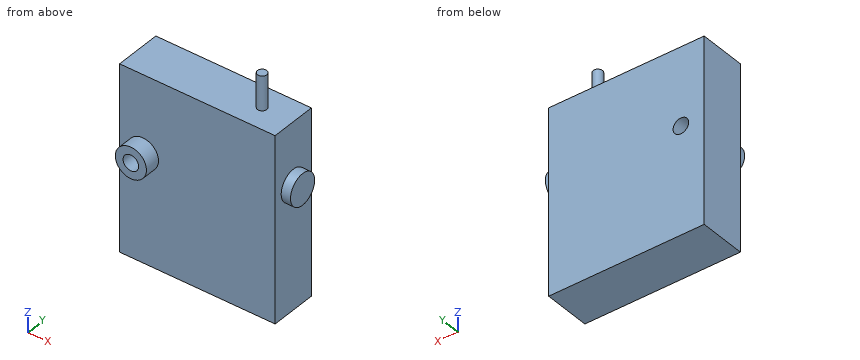
from build123d import *

# Parameters (mm, degrees)
F0_W     = 100
F0_H     = 119.065711
F1_DEPTH = 15
F2_R     = 10
F3_DEPTH = 10
F4_R     = 10
F5_DEPTH = 6
F6_R     = 3
F7_DEPTH = 22
F8_R     = 5
F9_DEPTH = 40.001


with BuildPart() as f1:
    # F0 (on Front) → F1 (new body, symmetric)
    with BuildSketch(Plane.XZ):
        with Locations((0, -3.62726)):
            Rectangle(F0_W, F0_H)
    extrude(amount=F1_DEPTH, both=True)

    # F2 (on face) → F3 (join)
    with BuildSketch(Plane.XZ.offset(15)):
        with Locations((-35, 5.905595)):
            Circle(F2_R)
    extrude(amount=F3_DEPTH)

    # F4 (on face) → F5 (join)
    with BuildSketch(Plane.YZ.offset(50)):
        with Locations((0, 15.905595)):
            Circle(F4_R)
    extrude(amount=F5_DEPTH)

    # F6 (on face) → F7 (join)
    with BuildSketch(Plane.XY.offset(55.905595)):
        with Locations((30, 0)):
            Circle(F6_R)
    extrude(amount=F7_DEPTH)

    # F8 (on face) → F9 (cut, through all)
    with BuildSketch(Plane.XZ.offset(25)):
        with Locations((-35, 5.905595)):
            Circle(F8_R)
    extrude(amount=-F9_DEPTH, mode=Mode.SUBTRACT)


solid = f1.part
Source: CAD feature listing. Evaluate the final solid. Frame: model axes, mm. Coordinates: 2 decimals unless noted, no trailing zeros. Order: outer loops, then holes, each group sorted by start corner. A loop starts at its lowest first (then second) coordinate and runs counter-clockwise, first axis right, second up. Notation, with made-up numbers: M 1,68.5 L 35,68.5 A24 cw 35,103.5 Z; hole C 30.25,14.5 d4. An arc over 180 degrees is marked long. Write each question's results on one line, items separated by ' | '. Start each with the question number.
1. Pin query (flat end, axial travel): pin 1 (4 mm diameter, centred on x = -34, y = -18.5, fed in from -Z); pin 2 (5 mm diameter, centred on x = -15, y = -9, fed in from +Z); pin 3 (6 mm diameter, centred on x = -35, z = 5.91, fed in from +Y); pin 4 (4 mm diameter, centred on y = -15.5, z = -47.5, fed in from +X). Return the tip coordinate at first contact, or that it passes through.
2. Section B-B, the plane y = 0. Return the cut outline in (x, z).
3. Section C-C, the plane x = 30. Return the cut outline in (y, z).
4. Section A-A, the plane x = -35. Return the cut outline in (y, z), then the cut area to 3 significant figures.
5. Material intervals for L1, parallel to Z at x = -35, y = 4.5; L2, parallel to Y at x = -12.5, z = 2; L3, parallel to Z at x = -25.5, y = -0.5, sorted ascending.
6. Section D-D, the plane z = 47.5. Return the cut outline in (x, y), then the cut area to 3 significant figures.
Solution:
1) pin 1: z = -4.09 | pin 2: z = 55.91 | pin 3: through | pin 4: x = 50
2) outline: M -50,-63.16 L 50,-63.16 L 50,5.91 L 56,5.91 L 56,25.91 L 50,25.91 L 50,55.91 L 33,55.91 L 33,77.91 L 27,77.91 L 27,55.91 L -50,55.91 Z; hole C -35,5.91 d10
3) outline: M -15,-63.16 L 15,-63.16 L 15,55.91 L 3,55.91 L 3,77.91 L -3,77.91 L -3,55.91 L -15,55.91 Z
4) outline: M -25,-4.09 L -15,-4.09 L -15,-63.16 L 15,-63.16 L 15,0.91 L -25,0.91 Z; M -25,10.91 L 15,10.91 L 15,55.91 L -15,55.91 L -15,15.91 L -25,15.91 Z | area: 3,370 mm²
5) L1: -63.16 to 0.91, 10.91 to 55.91 | L2: -15 to 15 | L3: -63.16 to 55.91
6) outline: M -50,-15 L 50,-15 L 50,15 L -50,15 Z | area: 3,000 mm²
